Work out the finished part from the listing and answer in its coordinate system (mm). Give positions to 0.01 mm unless a question says otherwise; leave off trailing zeros. Order: outer loops, then holes, each group sorted by start corner. A loop starts at its lowest first (then second) coordinate and runs counter-clockwise, first axis right, second up. Notation, with made-up numbers: (82, -19.5) -> (127, -19.5) arc R35 cw to (127, 18.5) -> close; hole circle Ø4 at (8.5, -22). An arc over 180 degrees is marked (long way). Answer as CSV lines item,"result". Start each with the question number.
1. Flat-ended cylindrical pins translate along their axes: pin 1 (5 mm diameter, centred on x = 324, y = 7, fed in from +Z); pin 2 (4 mm diameter, centred on x = 252, y = 4, fed in from -Z); pin 3 (3 mm diameter, centred on x = 123.5, y = 4.5, fed in from -Z). Find the tip coordinate at first contact, or state that the pin passes through.
2. Find the intervals of material crossed by L1, parallel to X at y = 6.75, z = 37.5; L2, parallel to X at y = 9, z = 60; L3, parallel to Z at x = 267, y = 9.5, in increasing order.
3. A cutting plane is placed at B-B (z = 86). Give the vertices of the cut face in (x, y), then the cut area to 3 significant figures.
4. A cutting plane is placed at A-A (y = 6). State how many separate pieces and enclosed holes the cut face has, then the cut area to 3 significant figures.
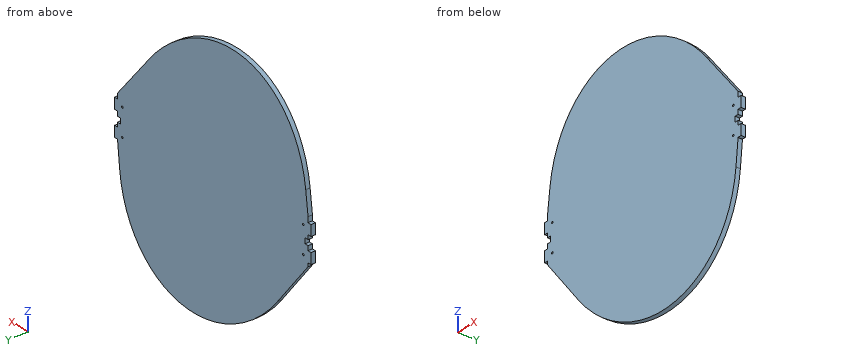
from build123d import *

# Parameters (mm, degrees)
BOSS_EXTRUDE1_DEPTH          = 12
SKETCH2_W                    = 10
SKETCH2_H                    = 15
CUT_EXTRUDE1_DEPTH           = 12
F_5_0_5_DIAMETER_HOLE2_D     = 5
F_5_0_5_DIAMETER_HOLE2_DEPTH = 25
F_5_0_5_DIAMETER_HOLE2_TIP   = 1.502151548


with BuildPart() as part:
    # Sketch1 → Boss-Extrude1 (new body)
    with BuildSketch(Plane(origin=(0, 0, 0), x_dir=(1, 0, 0), z_dir=(0, 1, 0))):
        with BuildLine():
            Line((-320, -65), (-312.170159719, -128.33520269))
            add(Edge.make_bspline(
                [(-312.170159719, -128.33520269), (-232.721291269, -770.993291043), (212.28214963, -202.588475219)],
                knots=[5.492316601, 5.492316601, 5.492316601, 7.67057167, 7.67057167, 7.67057167], degree=2, weights=[1, 0.463258742, 1]))
            Line((212.28214963, -202.588475219), (320, -65))
            Line((320, -65), (320, -50))
            Line((320, -50), (330, -50))
            Line((330, -50), (330, -20))
            Line((330, -20), (320, -20))
            Line((320, -20), (320, 20))
            Line((320, 20), (330, 20))
            Line((330, 20), (330, 50))
            Line((330, 50), (320, 50))
            Line((320, 50), (320, 51))
            Line((320, 51), (313.091302172, 120.09271769))
            add(Edge.make_bspline(
                [(313.091302172, 120.09271769), (244.337364097, 807.689215884), (-217.547896668, 195.738545202)],
                knots=[2.326299806, 2.326299806, 2.326299806, 4.55185667, 4.55185667, 4.55185667], degree=2, weights=[1, 0.442171166, 1]))
            Line((-217.547896668, 195.738545202), (-320, 60))
            Line((-320, 60), (-320, 50))
            Line((-320, 50), (-330, 50))
            Line((-330, 50), (-330, 20))
            Line((-330, 20), (-320, 20))
            Line((-320, 20), (-320, -20))
            Line((-320, -20), (-330, -20))
            Line((-330, -20), (-330, -50))
            Line((-330, -50), (-320, -50))
            Line((-320, -50), (-320, -65))
        make_face()
    extrude(amount=BOSS_EXTRUDE1_DEPTH)

    # Sketch2 → Cut-Extrude1 (cut)
    with BuildSketch(Plane.XZ):
        with Locations((315, 0)):
            Rectangle(SKETCH2_W, SKETCH2_H)
        with Locations((-315, 0)):
            Rectangle(SKETCH2_W, SKETCH2_H)
    extrude(amount=-CUT_EXTRUDE1_DEPTH, mode=Mode.SUBTRACT)

    # Ø5.0 (5) Diameter Hole2
    with Locations(Plane(origin=(0, -12, 0), x_dir=(-1, 0, 0), z_dir=(0, -1, 0))):
        with Locations((304, 37.5), (304, -37.5), (-304, -37.5), (-304, 37.5)):
            Hole(F_5_0_5_DIAMETER_HOLE2_D / 2, depth=F_5_0_5_DIAMETER_HOLE2_DEPTH)
            with Locations((0, 0, -(F_5_0_5_DIAMETER_HOLE2_DEPTH + F_5_0_5_DIAMETER_HOLE2_TIP / 2))):  # 118° drill point
                Cone(0, F_5_0_5_DIAMETER_HOLE2_D / 2, F_5_0_5_DIAMETER_HOLE2_TIP, mode=Mode.SUBTRACT)


solid = part.part
Answer sheet:
1,pin 1,"stops at z = 50"
1,pin 2,"stops at z = -278.62"
1,pin 3,"stops at z = -354.72"
2,L1,"x = -330 to -306.5, -301.5 to 301.5, 306.5 to 330"
2,L2,"x = -320 to 320"
2,L3,"z = -255.85 to 132.7"
3,outline,"(-317.4, 0) -> (303.56, 0) -> (303.56, 12) -> (-317.4, 12) -> close"
3,area,"7,450 mm^2"
4,separate pieces,"1"
4,enclosed holes,"4"
4,area,"354,000 mm^2"
